The model under review builds one solid part; all positions refer to its coordinate system, in mm. A direction names the side the tool comes from. Coordinates: 2 decimals unless noted, no trailing zeros. Write each loop counter-clockwise with the first axis right and the second up, starting at its lowest first coordinate (ties: lowest second). Pieces come first, ordered by that corner, then holes. Notation, with made-up numbers: (35.5, 31) -> (54.5, 31) arc R13 ccw to (54.5, 47) -> close; hole circle Ø1 at (-27.75, 2). An arc over 180 degrees is marked (long way). Put each result on its own line as item: value. Start each with the question number.
from build123d import *

# Parameters (mm, degrees)
F0_W     = 635
F0_H     = 558.8
F1_DEPTH = 6.35
F2_W     = 546.1
F2_H     = 393.7
F3_DEPTH = 158.75
F4_T     = -2.54
F2_R     = 25.4
F5_DEPTH = 25.4


with BuildPart() as f1:
    # F0 (on Top) → F1 (new body)
    with BuildSketch(Plane.XY):
        with Locations((-151.5700068397, -3.3926498145)):
            Rectangle(F0_W, F0_H)
    extrude(amount=F1_DEPTH)

    # F2 (on face) → F3 (join)
    with BuildSketch(Plane(origin=(0, 0, 0), x_dir=(1, 0, 0), z_dir=(0, 0, -1))):
        with Locations((-151.5700068397, 41.4926498145)):
            Rectangle(F2_W, F2_H)
    extrude(amount=F3_DEPTH)

    # F4
    f4_openings = [f1.faces().sort_by_distance(p)[0] for p in [
        (-151.570007, -3.39265, 6.35),
    ]]
    offset(amount=F4_T, openings=f4_openings, kind=Kind.INTERSECTION)

    # F2 (on face) → F5 (cut)
    with BuildSketch(Plane(origin=(0, 0, 0), x_dir=(1, 0, 0), z_dir=(0, 0, -1))):
        with Locations((-278.5700068397, -198.1609463692)):
            Circle(F2_R)
        with Locations((-151.5700068397, -198.1609463692)):
            Circle(F2_R)
        with Locations((-24.5700068397, -198.1609463692)):
            Circle(F2_R)
    extrude(amount=-F5_DEPTH, mode=Mode.SUBTRACT)


solid = f1.part
1. Consider section C-C on y = -66. State the section outline as (x, z) points, then the cut area to 3 significant figures.
2. Tool access review of faces 4 (the cylindrical face through (-30.076, 222.957, 1.252)), 5 (the flat face through (121.48, -39, -78)), 6 (the flat face through (-424.62, -39, -78)), 7 (the flat face through (-155, 155.357, -78)), 8 (the flat face through (118.94, -39, -76)): name each direction out of +Z, -Z, +X, -X, +Y, -Y from which nothing blocks a thin tool from reaching the whole face with its end or side.
3. Insertion check: P1, Ø12, axis at y = 95.5, z = -91, coming from the +X side; P2, Ø5, axis at x = -20.5, y = 108, coming from the +Z side; P3, Ø12, axis at y = -205, z = -136.5, coming from the -X side. Each pin has a flat end and moves straight along its axis. Give the tip position at first contact, or say it passes through.
4. Consider section D-D on x = -280.5. State the section outline as (y, z) points, then the cut area to 3 significant figures.
5. Consider section A-A on z = -143.5. State the section outline as (x, y) points.
6. The part is to be moulded in two halves that separate along Y. For faces 1 (the flat face through (-422.08, -39, -76)), 2 (the flat face through (-155, -238.343, -78)), 3 (the flat face through (-155, -44, -158.75)), say which applies: released by +Y, released by -Y, zero draft, split by the parting line, or undercut.
7. Wall thickness on line 1 (Y direction, x = 23.5, z = -44); line 2 (X direction, y = 93, z = -23); line 3 (Z direction, x = -304, y = 115.5): over which ranges is each line inside the solid? List them lowest first. Write a range as from..to.
8. Consider section B-B on x = -385. State the section outline as (y, z) points.
Output values:
1. outline: (-469.07, 0) -> (-424.62, 0) -> (-424.62, -158.75) -> (121.48, -158.75) -> (121.48, 0) -> (165.93, 0) -> (165.93, 6.35) -> (163.39, 6.35) -> (163.39, 2.54) -> (118.94, 2.54) -> (118.94, -156.21) -> (-422.08, -156.21) -> (-422.08, 2.54) -> (-466.53, 2.54) -> (-466.53, 6.35) -> (-469.07, 6.35) -> close
1. area: 2,440 mm^2
2. face 4: +Z, -Z
2. face 5: -Z, +X, +Y, -Y
2. face 6: -Z, -X, +Y, -Y
2. face 7: -Z, +X, -X, +Y
2. face 8: +Z
3. P1: stops at x = 121.48
3. P2: stops at z = -156.21
3. P3: stops at x = -424.62
4. outline: (-282.79, 0) -> (-238.34, 0) -> (-238.34, -158.75) -> (155.36, -158.75) -> (155.36, 0) -> (172.83, 0) -> (172.83, 2.54) -> (152.82, 2.54) -> (152.82, -156.21) -> (-235.8, -156.21) -> (-235.8, 2.54) -> (-280.25, 2.54) -> (-280.25, 6.35) -> (-282.79, 6.35) -> close; (223.49, 0) -> (276.01, 0) -> (276.01, 6.35) -> (273.47, 6.35) -> (273.47, 2.54) -> (223.49, 2.54) -> close
4. area: 2,120 mm^2
5. outline: (-424.62, -238.34) -> (121.48, -238.34) -> (121.48, 155.36) -> (-424.62, 155.36) -> close; hole (-422.08, -235.8) -> (118.94, -235.8) -> (118.94, 152.82) -> (-422.08, 152.82) -> close
6. face 1: undercut
6. face 2: released by -Y
6. face 3: zero draft
7. line 1: y = -238.34..-235.8, 152.82..155.36
7. line 2: x = -424.62..-422.08, 118.94..121.48
7. line 3: z = -158.75..-156.21
8. outline: (-282.79, 0) -> (-238.34, 0) -> (-238.34, -158.75) -> (155.36, -158.75) -> (155.36, 0) -> (276.01, 0) -> (276.01, 6.35) -> (273.47, 6.35) -> (273.47, 2.54) -> (152.82, 2.54) -> (152.82, -156.21) -> (-235.8, -156.21) -> (-235.8, 2.54) -> (-280.25, 2.54) -> (-280.25, 6.35) -> (-282.79, 6.35) -> close
